Design review of the part built by this model. Coordinates are the model's own, in mm. A direction names the side the tool comes from. Give positions to 0.01 mm unless a question says otherwise; leave off trailing zeros. Order: outer loops, then holes, each group sorted by start corner. A loop starts at its lowest first (then second) coordinate and runs counter-clockwise, first axis right, second up. Notation, with made-up numbers: M -23.75,37 L -19.75,37 A17 ccw -19.75,63 Z; hole C -0.75,-3 d6. An arc over 180 degrees is marked long. Answer as a JSON object with one key per item and string values.
from build123d import *

# Parameters (mm, degrees)
CYLINDER001_R     = 4.05
CYLINDER001_DEPTH = 28
CYLINDER_R        = 6
CYLINDER_DEPTH    = 21
SKETCH_R          = 7
PAD_DEPTH         = 2
CHAMFER_SIZE      = 0.99
CHAMFER001_SIZE   = 1
CHAMFER002_SIZE   = 0.5


with BuildPart() as cilindro001:
    # Cylinder001 → Cylinder001 (new body)
    with BuildSketch(Plane.XY.offset(-1)):
        Circle(CYLINDER001_R)
    extrude(amount=CYLINDER001_DEPTH)


with BuildPart() as chamfer002:
    # Cylinder → Cylinder (new body)
    with BuildSketch(Plane.XY):
        Circle(CYLINDER_R)
    extrude(amount=CYLINDER_DEPTH)

    # Sketch → Pad (new body)
    with BuildSketch(Plane.XY.offset(21)):
        Circle(SKETCH_R)
    extrude(amount=PAD_DEPTH)

    # Cut: cut Cilindro001
    add(cilindro001.part, mode=Mode.SUBTRACT)

    # Chamfer
    chamfer_edges = [chamfer002.edges().sort_by_distance(p)[0] for p in [
        (-6, 0, 21),
    ]]
    chamfer(chamfer_edges, length=CHAMFER_SIZE)

    # Chamfer001
    chamfer001_edges = [chamfer002.edges().sort_by_distance(p)[0] for p in [
        (-6, 0, 0),
    ]]
    chamfer(chamfer001_edges, length=CHAMFER001_SIZE)

    # Chamfer002
    chamfer002_edges = [chamfer002.edges().sort_by_distance(p)[0] for p in [
        (-4.05, 0, 23),
    ]]
    chamfer(chamfer002_edges, length=CHAMFER002_SIZE)


solid = chamfer002.part
(1) Tool access review of faces 4 (the cylindrical face through (-6, 0, 10)), 5 (the flat face through (2, -4, 0)): name each direction out of +Z, -Z, +X, -X, +Y, -Y from which nothing blocks a thin tool from reaching the whole face with its end or side.
Checked values:
{"face 4": "-Z", "face 5": "-Z, +X, -X, +Y, -Y"}
(2) Draft analysis for pull direction Y (two halves, no side actions). For faces 1 (the cylindrical face through (6.466, -2.681, 21.986)), 2 (the cylindrical face through (-0.878, -3.954, 11.092)), 3 (the flat face through (0, -5, 23)), state which applies: +Y half, -Y half, draft (parallel to the pull), parting line (faces both ways), or undercut.
Checked values:
{"face 1": "parting line", "face 2": "undercut", "face 3": "draft"}
(3) Insertion check: pin 1 (5 mm diameter, centred on y = 4.5, z = 15, fed in from +X); pin 2 (1.5 mm diameter, centred on x = 2, z = 11.5, fed in from +Y); pin 3 (1.5 mm diameter, centred on y = 4.5, z = 20.5, fed in from +X). Each pin has a flat end and moves straight along its axis. Give the tip position at first contact, or say it passes through.
Checked values:
{"pin 1": "stops at x = 5.66", "pin 2": "stops at y = 5.87", "pin 3": "stops at x = 5.79"}
(4) We need section C-C (z = 14.5). Write out the cut boundary in (x, y).
Checked values:
{"outline": "C 0,0 d12; hole C 0,0 d8.1"}
(5) To check wall thickness, follow L1, parallel to Y at x = 0, z = 5; L2, parallel to Y at x = -1, z = 11.5; L3, parallel to X at y = -1.75, z = 15.25. State the ranges of each line that lie inside material, in increasing order. Write a range as from..to.
Checked values:
{"L1": "y = -6..-4.05, 4.05..6", "L2": "y = -5.92..-3.92, 3.92..5.92", "L3": "x = -5.74..-3.65, 3.65..5.74"}
